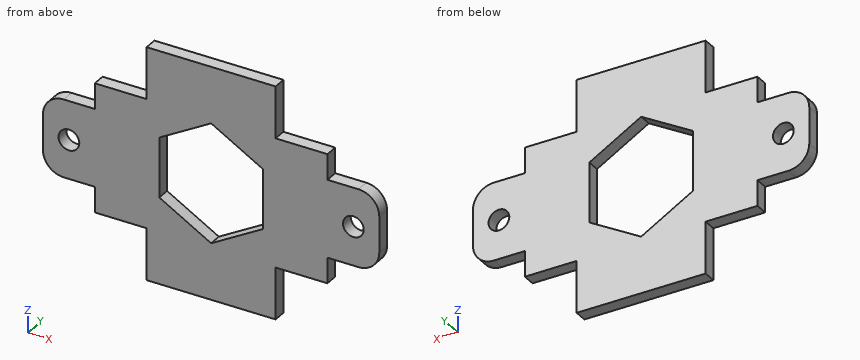
from build123d import *

# Parameters (mm, degrees)
SKETCH1_R           = 2.54
BOSS_EXTRUDE1_DEPTH = 3.175


with BuildPart() as part:
    # Sketch1 → Boss-Extrude1 (new body)
    with BuildSketch(Plane(origin=(0, 0, 0), x_dir=(1, 0, 0), z_dir=(0, 1, 0))):
        with BuildLine():
            Line((-28.4999938, 15.7999938), (-28.4999938, 9.525))
            Line((-28.4999938, 9.525), (-36.1199938, 9.525))
            ThreePointArc((-36.1199938, 9.525), (-39.712096248, 8.037102448), (-41.1999938, 4.445))
            Line((-41.1999938, 4.445), (-41.1999938, -4.445))
            ThreePointArc((-41.1999938, -4.445), (-39.712096248, -8.037102448), (-36.1199938, -9.525))
            Line((-36.1199938, -9.525), (-28.4999938, -9.525))
            Line((-28.4999938, -9.525), (-28.4999938, -15.7999938))
            Line((-28.4999938, -15.7999938), (-15.7999938, -15.7999938))
            Line((-15.7999938, -15.7999938), (-15.7999938, -28.4999938))
            Line((-15.7999938, -28.4999938), (15.7999938, -28.4999938))
            Line((15.7999938, -28.4999938), (15.7999938, -15.7999938))
            Line((15.7999938, -15.7999938), (28.4999938, -15.7999938))
            Line((28.4999938, -15.7999938), (28.4999938, -9.525))
            Line((28.4999938, -9.525), (36.1199938, -9.525))
            ThreePointArc((36.1199938, -9.525), (39.712096248, -8.037102448), (41.1999938, -4.445))
            Line((41.1999938, -4.445), (41.1999938, 4.445))
            ThreePointArc((41.1999938, 4.445), (39.712096248, 8.037102448), (36.1199938, 9.525))
            Line((36.1199938, 9.525), (28.4999938, 9.525))
            Line((28.4999938, 9.525), (28.4999938, 15.7999938))
            Line((28.4999938, 15.7999938), (15.7999938, 15.7999938))
            Line((15.7999938, 15.7999938), (15.7999938, 28.4999938))
            Line((15.7999938, 28.4999938), (-15.7999938, 28.4999938))
            Line((-15.7999938, 28.4999938), (-15.7999938, 15.7999938))
            Line((-15.7999938, 15.7999938), (-28.4999938, 15.7999938))
        make_face()
        with Locations((-34.8499938, 0)):
            Circle(SKETCH1_R, mode=Mode.SUBTRACT)
        with Locations((34.8499938, 0)):
            Circle(SKETCH1_R, mode=Mode.SUBTRACT)
        Polygon((0, 14.664696837), (-12.7, 7.332348419), (-12.7, -7.332348419), (0, -14.664696837), (12.7, -7.332348419), (12.7, 7.332348419), align=None, mode=Mode.SUBTRACT)
    extrude(amount=BOSS_EXTRUDE1_DEPTH)


solid = part.part
Geometry: final body of the model. Coordinates: model frame, mm. Give positions to 0.01 mm unless a question says otherwise; leave off trailing zeros. Write each loop counter-clockwise with the first axis right and the second up, starting at its lowest first coordinate (ties: lowest second). Pieces come first, ordered by that corner, then holes. Notation, with made-up numbers: (0, 79) -> (42, 79) arc R30 ccw to (42, 116) -> close; hole circle Ø8 at (-1.5, -10). An arc over 180 degrees is marked (long way). Answer in a Markdown table with one row per item.
(1) Section query C-C on z = 23.5. Return loops of the section in (x, y) (3 decimals), then the cut area to 3 significant figures.
Answers below:
| item | result |
|---|---|
| outline | (-15.8, 0) -> (15.8, 0) -> (15.8, 3.175) -> (-15.8, 3.175) -> close |
| area | 100 mm^2 |
(2) Section query D-D on x = -23. Return loops of the section in (y, z) (3 decimals), then the cut area to 3 significant figures.
Answers below:
| item | result |
|---|---|
| outline | (0, -15.8) -> (3.175, -15.8) -> (3.175, 15.8) -> (0, 15.8) -> close |
| area | 100 mm^2 |
(3) Ray query, line 1 along X through (y, z) = (1.7, 0); line 2 along X through (y, z) = (2.2, 2); line 3 along X through (y, z) = (0.7, -4.5). Return the intervals inside material, ascending. Write a range as [from, to].
Answers below:
| item | result |
|---|---|
| line 1 | [-41.2, -37.39], [-32.31, -12.7], [12.7, 32.31], [37.39, 41.2] |
| line 2 | [-41.2, -36.42], [-33.28, -12.7], [12.7, 33.28], [36.42, 41.2] |
| line 3 | [-41.2, -12.7], [12.7, 41.2] |
(4) Section query A-A on z = 0. Return loops of the section in (x, y) (3 decimals), then the cut area to 3 significant figures.
Answers below:
| item | result |
|---|---|
| outline | (-41.2, 0) -> (-37.39, 0) -> (-37.39, 3.175) -> (-41.2, 3.175) -> close; (-32.31, 0) -> (-12.7, 0) -> (-12.7, 3.175) -> (-32.31, 3.175) -> close; (12.7, 0) -> (32.31, 0) -> (32.31, 3.175) -> (12.7, 3.175) -> close; (37.39, 0) -> (41.2, 0) -> (41.2, 3.175) -> (37.39, 3.175) -> close |
| area | 149 mm^2 |
(5) Section query B-B on y = 2.05. State how many separate pieces and enclosed holes the cut face has, then the cut area to 3 significant figures.
Answers below:
| item | result |
|---|---|
| separate pieces | 1 |
| enclosed holes | 3 |
| area | 2,470 mm^2 |
(6) Pin query (flat end, axial travel): pin 1 (1 mm diameter, centred on y = 2, z = 19.5, fed in from -X); pin 2 (6 mm diameter, centred on x = 34.85, z = 0, fed in from -Y); pin 3 (1 mm diameter, centred on y = 2, z = 24, fed in from +X); pin 4 (1.6 mm diameter, centred on y = 1.5, z = -12.5, fed in from +X). Return the tip coordinate at first contact, or that it passes through.
Answers below:
| item | result |
|---|---|
| pin 1 | x = -15.8 |
| pin 2 | y = 0 |
| pin 3 | x = 15.8 |
| pin 4 | x = 28.5 |
